Input: part model. Units: mm. Frame: model coordinates. Face numbers are marked on the shaded views. A direction names the side the tool comes from. Give positions to 0.01 mm unless a question says otherwise; leave off trailing zeros. Order: outer loops, then holes, each group sorted by start corner. A loop starts at its lowest first (then second) coordinate and runs counter-clockwise, first axis right, second up. Notation, with made-up numbers: (15, 81) - (41, 81) arc R22 ccw to (41, 101) - close; hole circle Ø10 at (-29, 26). An arc over 180 degrees is marked (long way). Answer in a Markdown table with one row per item. Add a question column.
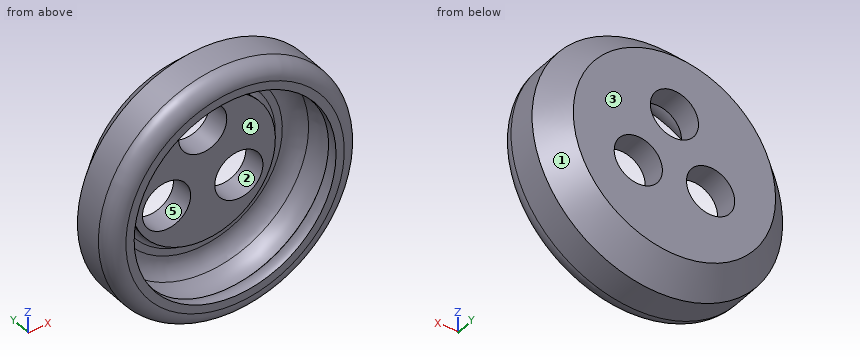
from build123d import *

# Parameters (mm, degrees)
CUT_EXTRUDE1_REACH = 24.772
SKETCH3_R          = 3


with BuildPart() as part:
    # Sketch2 → Revolve1 (revolve)
    with BuildSketch(Plane.XY, mode=Mode.PRIVATE) as revolve1_sk:
        with BuildLine():
            Line((-12.593114148, 22.177254176), (-15.593114148, 19.177254176))
            Line((-15.593114148, 19.177254176), (-15.593114148, 15.495111766))
            ThreePointArc((-15.593114148, 15.495111766), (-15.00732771, 14.080898204), (-13.593114148, 13.495111766))
            Line((-13.593114148, 13.495111766), (-12.565328021, 13.495111766))
            ThreePointArc((-12.565328021, 13.495111766), (-12.634939156, 14.785886966), (-13.41748538, 15.814754176))
            ThreePointArc((-13.41748538, 15.814754176), (-13.513613389, 15.897930793), (-13.593114148, 15.997120375))
            ThreePointArc((-13.593114148, 15.997120375), (-13.503619616, 17.46180735), (-12.915716215, 18.806309784))
            ThreePointArc((-12.915716215, 18.806309784), (-11.959555448, 19.80834635), (-10.624554433, 20.177254176))
            Line((-10.624554433, 20.177254176), (-9.75, 20.177254176))
            ThreePointArc((-9.75, 20.177254176), (-9.255025253, 19.972228922), (-9.05, 19.477254176))
            Line((-9.05, 19.477254176), (-9.05, 19.177254176))
            Line((-9.05, 19.177254176), (0, 19.177254176))
            Line((0, 19.177254176), (0, 22.177254176))
            Line((0, 22.177254176), (-12.593114148, 22.177254176))
        make_face()
    revolve(revolve1_sk.sketch.rotate(Axis((0, 0, 0), (0, 1, 0)), 270), axis=Axis((0, 0, 0), (0, 1, 0)))

    # Sketch3 → Cut-Extrude1 (cut, up to next)
    with BuildSketch(Plane.XZ.offset(-19.177254176), mode=Mode.PRIVATE) as cut_extrude1_sk1:
        with Locations(Location((-4.5, -2.598076211, 0), (0, 0, 270))):
            Circle(SKETCH3_R)
    cut_extrude1_tool1 = extrude(cut_extrude1_sk1.sketch, amount=-CUT_EXTRUDE1_REACH, mode=Mode.PRIVATE) & part.part
    # Sketch3 → Cut-Extrude1 (cut, up to next)
    with BuildSketch(Plane.XZ.offset(-19.177254176), mode=Mode.PRIVATE) as cut_extrude1_sk2:
        with Locations(Location((4.5, -2.598076211, 0), (0, 0, 270))):
            Circle(SKETCH3_R)
    cut_extrude1_tool2 = extrude(cut_extrude1_sk2.sketch, amount=-CUT_EXTRUDE1_REACH, mode=Mode.PRIVATE) & part.part
    # Sketch3 → Cut-Extrude1 (cut, up to next)
    with BuildSketch(Plane.XZ.offset(-19.177254176), mode=Mode.PRIVATE) as cut_extrude1_sk3:
        with Locations(Location((0, 5.196152423, 0), (0, 0, 270))):
            Circle(SKETCH3_R)
    cut_extrude1_tool3 = extrude(cut_extrude1_sk3.sketch, amount=-CUT_EXTRUDE1_REACH, mode=Mode.PRIVATE) & part.part
    add(cut_extrude1_tool1.solids().sort_by_distance((-4.5, 19.177254, -2.598076))[0], mode=Mode.SUBTRACT)
    add(cut_extrude1_tool2.solids().sort_by_distance((4.5, 19.177254, -2.598076))[0], mode=Mode.SUBTRACT)
    add(cut_extrude1_tool3.solids().sort_by_distance((0, 19.177254, 5.196152))[0], mode=Mode.SUBTRACT)


solid = part.part
Q1. Pull-direction query (Z, two-part tool) for the marked faces 1, 2 and 3; classes: +Z half, -Z half, draft (parallel to the pull), parting line (faces both ways), or undercut.
Q2. Line query: probe 1 along X at (y, z) = (16.5, 11); probe 2 along X at (y, z) = (17, 6); probe 3 along Y at (x, z) = (8, -10). Output: solid intervals per line, ascending.
Q3. Access query for the marked faces 4 and 5. Directions: +Z, -Z, +X, -X, +Y, -Y. A direction counts if a zero-diameter tool reaches every point of the face in a straight line with its end or side. Return the directions, or none.
Q4. Contact query for flat-ended pins moving along their axis: P1, Ø8, axis at x = 4.5, z = -2.6, coming from the -Y side; P2, Ø5, axis at x = -4.5, z = -2.6, coming from the +Y side (1 decimal); P3, Ø2, axis at x = -11, y = 20.5, coming from the -Z side; P4, Ø4, axis at y = 14.5, z = -6, coming from the -X side. Output: stop coordinate, or through.
Q5. Section A-A, the plane z = 0. State how many separate pieces and enclosed holes the cut face has, then the cut area to 3 significant figures.
Q6. Section B-B, the plane y = 18.25. Return loops of the section in (x, z), then the cut area to 3 significant figures.
Computed:
| question | item | result |
|---|---|---|
| 1 | face 1 | parting line |
| 1 | face 2 | undercut |
| 1 | face 3 | draft |
| 2 | probe 1 | x = -11.05 to -8.03, 8.03 to 11.05 |
| 2 | probe 2 | x = -14.39 to -12.19, 12.19 to 14.39 |
| 2 | probe 3 | y = 13.5 to 15.15, 18.99 to 21.96 |
| 3 | face 4 | -Y |
| 3 | face 5 | +Y, -Y |
| 4 | P1 | stops at y = 19.18 |
| 4 | P2 | passes through |
| 4 | P3 | stops at z = -10.91 |
| 4 | P4 | stops at x = -15.02 |
| 5 | separate pieces | 3 |
| 5 | enclosed holes | 0 |
| 5 | area | 87.4 mm^2 |
| 6 | outline | circle Ø31.19 at (0, 0); hole circle Ø26.46 at (0, 0) |
| 6 | area | 214 mm^2 |
